Read the model definition and answer for the solid it produces. Units are mm, in the model's axes. A direction names the side the tool comes from. Coordinates: 2 decimals unless noted, no trailing zeros. Loops run counter-clockwise (first coordinate to the right, second up) from the corner with the lowest first, then second, coordinate; pieces in that order, holes last.
from build123d import *

# Parameters (mm, degrees)
SKETCH1_R           = 11
BOSS_EXTRUDE1_DEPTH = 20
SKETCH2_R           = 10
CUT_EXTRUDE1_DEPTH  = 18
FILLET1_R           = 1
CUT_EXTRUDE2_REACH  = 27.338
SKETCH3_R           = 4


with BuildPart() as part:
    # Sketch1 → Boss-Extrude1 (new body)
    with BuildSketch(Plane(origin=(0, 0, 0), x_dir=(1, 0, 0), z_dir=(0, 1, 0))):
        with Locations(Location((0, 0, 0), (0, 0, 270))):
            Circle(SKETCH1_R)
    extrude(amount=BOSS_EXTRUDE1_DEPTH)

    # Sketch2 → Cut-Extrude1 (cut)
    with BuildSketch(Plane(origin=(0, 20, 0), x_dir=(1, 0, 0), z_dir=(0, 1, 0))):
        with Locations(Location((0, 0, 0), (0, 0, 270))):
            Circle(SKETCH2_R)
    extrude(amount=-CUT_EXTRUDE1_DEPTH, mode=Mode.SUBTRACT)

    # Fillet1
    fillet1_edges = [part.edges().sort_by_distance(p)[0] for p in [
        (0, 0, -11),
    ]]
    fillet(fillet1_edges, radius=FILLET1_R)

    # Sketch3 → Cut-Extrude2 (cut, up to next)
    with BuildSketch(Plane.XZ, mode=Mode.PRIVATE) as cut_extrude2_sk1:
        with Locations(Location((0, 0, 0), (0, 0, 270))):
            Circle(SKETCH3_R)
    cut_extrude2_tool1 = extrude(cut_extrude2_sk1.sketch, amount=-CUT_EXTRUDE2_REACH, mode=Mode.PRIVATE) & part.part
    add(cut_extrude2_tool1.solids().sort_by_distance((0, 0, 0))[0], mode=Mode.SUBTRACT)


solid = part.part
Item 1: A cutting plane is placed at A-A on x = 0. Determine the outline of the cut face in (y, z), then the cut area to 3 significant figures.
Numbers:
outline: (0, -10) arc R1 ccw to (1, -11) - (20, -11) - (20, -10) - (2, -10) - (2, -4) - (0, -4) - close; (0, 4) - (2, 4) - (2, 10) - (20, 10) - (20, 11) - (1, 11) arc R1 ccw to (0, 10) - close
area: 63.6 mm2
Item 2: A cutting plane is placed at C-C on y = 10.25. Determine the outline of the cut face in (x, z).
Numbers:
outline: circle Ø22 at (0, 0); hole circle Ø20 at (0, 0)
Item 3: Which of the six approach directions +Z, -Z, +X, -X, +Y, -Y give full straight-line access (tool end or side, diameter ignored) to faces 4 (the face through (0.1, 2, 4.3)), 5 (the face through (-3.905, 0.986, 0.867))?
Numbers:
face 4: +Y
face 5: +Y, -Y
Item 4: A cutting plane is placed at B-B on z = 0. Determine the outline of the cut face in (x, y), then the cut area to 3 significant figures.
Numbers:
outline: (-11, 1) arc R1 ccw to (-10, 0) - (-4, 0) - (-4, 2) - (-10, 2) - (-10, 20) - (-11, 20) - close; (4, 0) - (10, 0) arc R1 ccw to (11, 1) - (11, 20) - (10, 20) - (10, 2) - (4, 2) - close
area: 63.6 mm2
Item 5: Find the intervals of material crossed by line 1 along X through (y, z) = (7.5, -0.25); line 2 along X through (y, z) = (1, 0); line 3 along Y through (x, z) = (6, 1), in increasing order.
Numbers:
line 1: x = -11 to -10, 10 to 11
line 2: x = -11 to -4, 4 to 11
line 3: y = 0 to 2
Item 6: Determine the mould class of faces 1 (the face through (-9.76, 11.13, -2.17)), 2 (the face through (-10.74, 10.37, -2.38)), 3 (the face through (-10, 20, 2)) for opening direction X: released by +X, released by -X, zero draft, split by the parting line, or undercut.
Numbers:
face 1: undercut
face 2: split by the parting line
face 3: zero draft
Item 7: Given pin 1 (1.5 mm diameter, centred on x = -4, z = 1.5, fed in from +Y); pin 2 (5 mm diameter, centred on y = 13, z = -3, fed in from +X); pin 3 (3 mm diameter, centred on x = -2, y = 15, fed in from -Z), each flat-ended and moving along its own axis, determine where each tip first touches the part or whether it passes through.
Numbers:
pin 1: stops at y = 2
pin 2: stops at x = 10.99
pin 3: stops at z = -10.99
